Model file for the job. Use its own axes, mm. Give positions to 0.01 mm unless a question says otherwise; leave off trailing zeros. Loops run counter-clockwise (first coordinate to the right, second up) from the corner with the lowest first, then second, coordinate; pieces in that order, holes last. Notation, with made-up numbers: M -9.5,-5.75 L 13.5,-5.75 A33 cw 13.5,27.25 Z; hole C 4,76 d3. An arc over 180 degrees is marked long. Answer in a Markdown table with one row per item.
```python
from build123d import *

# Parameters (mm, degrees)
EXTRUDE_1_DEPTH                = 5
SKETCH_2_R                     = 13.5
CUT_EXTRUDE_1_DEPTH            = 5
SKETCH_4_R                     = 2.25
CUT_EXTRUDE_2_DEPTH            = 5
HOLE_WIZARD_M2_5_1_D           = 2.9
HOLE_WIZARD_M2_5_1_CBORE_D     = 5.5
HOLE_WIZARD_M2_5_1_CBORE_DEPTH = 2.5


with BuildPart() as part:
    # 스케치1 → 보스-돌출1 (new body)
    with BuildSketch(Plane(origin=(0, 0, 0), x_dir=(1, 0, 0), z_dir=(0, 1, 0))):
        with BuildLine():
            Line((-27.5, 15), (-27.5, -10))
            ThreePointArc((-27.5, -10), (0, -37.5), (27.5, -10))
            Line((27.5, -10), (27.5, 15))
            ThreePointArc((27.5, 15), (0, 42.5), (-27.5, 15))
        make_face()
    extrude(amount=EXTRUDE_1_DEPTH)

    # 스케치2 → 컷-돌출1 (cut)
    with BuildSketch(Plane(origin=(0, 5, 0), x_dir=(1, 0, 0), z_dir=(0, 1, 0))):
        with Locations((0, 17.5)):
            Circle(SKETCH_2_R)
    extrude(amount=-CUT_EXTRUDE_1_DEPTH, mode=Mode.SUBTRACT)

    # 스케치4 → 컷-돌출2 (cut)
    with BuildSketch(Plane(origin=(0, 5, 0), x_dir=(1, 0, 0), z_dir=(0, 1, 0))):
        with Locations((0, 37.5)):
            Circle(SKETCH_4_R)
        with Locations((0, -32.5)):
            Circle(SKETCH_4_R)
        with Locations((-22, 17.5)):
            Circle(SKETCH_4_R)
        with Locations((22, 17.5)):
            Circle(SKETCH_4_R)
    extrude(amount=-CUT_EXTRUDE_2_DEPTH, mode=Mode.SUBTRACT)

    # M2.5 소켓 머리 캡 나사용 카운터보어1 (through all)
    with Locations(Plane(origin=(0, 5, 0), x_dir=(1, 0, 0), z_dir=(0, 1, 0))):
        with Locations((-13.5, 28), (13.5, 28), (13.5, -24), (-13.5, -24)):
            CounterBoreHole(HOLE_WIZARD_M2_5_1_D / 2, HOLE_WIZARD_M2_5_1_CBORE_D / 2, HOLE_WIZARD_M2_5_1_CBORE_DEPTH)


solid = part.part
```
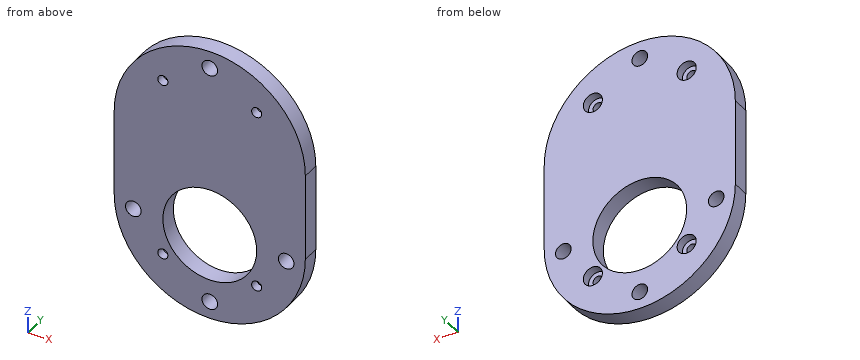
(1) Saw through at C-C, the plane z = -37.5. Give the cut face in (x, y), and give its area (3 significant figures).
Established:
| item | result |
|---|---|
| outline | M -15.81,0 L -2.25,0 L -2.25,5 L -15.81,5 Z; M 2.25,0 L 15.81,0 L 15.81,5 L 2.25,5 Z |
| area | 136 mm2 |
(2) Flat gauge pins, fed straight in: P1, Ø1.5, axis at x = 17, y = 3, coming from the -Z side; P2, Ø2.5, axis at x = 13.5, z = 24, coming from the -Y side; P3, Ø5, axis at x = -13.5, z = -28, coming from the +Y side; P4, Ø1, axis at x = -15, y = 4.5, coming from the +Z side. Where does each tip first touch, or does it go through?
Established:
| item | result |
|---|---|
| P1 | stops at z = -37.19 |
| P2 | passes through |
| P3 | stops at y = 2.5 |
| P4 | stops at z = 33.37 |
(3) Wall check: L1, parallel to Z at x = 0, y = 1.55; L2, parallel to Z at x = -1.5, y = 0.95; L3, parallel to X at y = 4.4, z = 24. Give the ranges that are in metal, low to high.
Established:
| item | result |
|---|---|
| L1 | z = -42.5 to -39.75, -35.25 to -31, -4 to 30.25, 34.75 to 37.5 |
| L2 | z = -42.46 to -39.18, -35.82 to -30.92, -4.08 to 30.82, 34.18 to 37.46 |
| L3 | x = -23.67 to -16.25, -10.75 to 10.75, 16.25 to 23.67 |
(4) Saw through at B-B, the plane y = 3.35. Count the separate pieces of the cut face and the enclosed holes in it, and give its area (3 significant figures).
Established:
| item | result |
|---|---|
| separate pieces | 1 |
| enclosed holes | 9 |
| area | 3,020 mm2 |
(5) Saw through at A-A, the plane x = -22. Give the cut face in (y, z).
Established:
| item | result |
|---|---|
| outline | M 0,-31.5 L 5,-31.5 L 5,-19.75 L 0,-19.75 Z; M 0,-15.25 L 5,-15.25 L 5,26.5 L 0,26.5 Z |
(6) Saw through at D-D, the plane z = -28. Give the cut face in (x, y).
Established:
| item | result |
|---|---|
| outline | M -24.23,0 L -14.95,0 L -14.95,2.5 L -16.25,2.5 L -16.25,5 L -24.23,5 Z; M -12.05,0 L -8.49,0 L -8.49,5 L -10.75,5 L -10.75,2.5 L -12.05,2.5 Z; M 8.49,0 L 12.05,0 L 12.05,2.5 L 10.75,2.5 L 10.75,5 L 8.49,5 Z; M 14.95,0 L 24.23,0 L 24.23,5 L 16.25,5 L 16.25,2.5 L 14.95,2.5 Z |
